```python
from build123d import *

# Parameters (mm, degrees)
CUT_EXTRUDE1_DEPTH       = 31.174758882
BOSS_EXTRUDE1_START      = 13.11
BOSS_EXTRUDE1_OUTLINE_R  = 7.478502705
BOSS_EXTRUDE1_DEPTH      = 10.08
CIRPATTERN1_COUNT        = 3
BOSS_EXTRUDE2_DEPTH      = 10.08
BOSS_EXTRUDE2_DEPTH_BACK = 495
SKETCH6_R                = 12.5


# Read off the part's stored shape, not the designer's step: Boss-Extrude1, Revolve3
with BuildPart() as part:
    # Sketch1 → Revolve1 (revolve)
    with BuildSketch(Plane.XY):
        with BuildLine():
            Line((-9.722222222, 14.550889837), (-9.722222222, 12.5))
            Line((-9.722222222, 12.5), (7.540919832, 12.5))
            Line((7.540919832, 12.5), (7.540919832, 15.791913376))
            ThreePointArc((7.540919832, 15.791913376), (-1.254812689, 17.454954744), (-9.722222222, 14.550889837))
        make_face()
    revolve(axis=Axis((-47.061566383, 0, 0), (1, 0, 0)))

    # Sketch2 → Cut-Extrude1 (cut, symmetric)
    with BuildSketch(Plane(origin=(7.540919832, 0, 0), x_dir=(0, 0, -1), z_dir=(1, 0, 0))):
        Polygon((-17.183661108, 13.11), (20.1337897, 13.11), (18.772985043, 23.764289573), (-17.183661108, 23.764289573), align=None)
    cut_extrude1 = extrude(amount=CUT_EXTRUDE1_DEPTH, both=True, mode=Mode.SUBTRACT)

    # Boss-Extrude1 outline → Boss-Extrude1 (add)
    with BuildSketch(Plane(origin=(0, 0, 0), x_dir=(1, 0, 0), z_dir=(0, 1, 0)).offset(BOSS_EXTRUDE1_START)):
        Circle(BOSS_EXTRUDE1_OUTLINE_R)
    boss_extrude1 = extrude(amount=BOSS_EXTRUDE1_DEPTH)

    # Sketch4 → Revolve2 (revolve)
    with BuildSketch(Plane(origin=(0, 0, 0), x_dir=(0, 0, -1), z_dir=(1, 0, 0)), mode=Mode.PRIVATE) as revolve2_sk:
        with BuildLine():
            Line((7.478502705, 25.422863672), (7.478502705, 23.19))
            Line((7.478502705, 23.19), (0, 23.19))
            Line((0, 23.19), (0, 26.5))
            ThreePointArc((0, 26.5), (3.777837522, 26.229333649), (7.478502705, 25.422863672))
        make_face()
    revolve2 = revolve(revolve2_sk.sketch.rotate(Axis((0, 0, 0), (0, 1, 0)), 180), axis=Axis((0, 0, 0), (0, 1, 0)))

    # Revolve3 outline → Revolve3 (revolve)
    with BuildSketch(Plane.XY):
        with BuildLine():
            Line((7.478502705, 23.190000012), (7.478502705, 13.109999988))
            Line((7.478502705, 13.109999988), (12.254015665, 13.109999994))
            ThreePointArc((12.254015665, 13.109999994), (13.25, 18.15), (12.254015665, 23.190000006))
            Line((12.254015665, 23.190000006), (7.478502705, 23.190000012))
        make_face()
    revolve3 = revolve(axis=Axis((0, 0, 0), (0, 1, 0)))

    # CirPattern1: Cut-Extrude1, Boss-Extrude1, Revolve2, Revolve3 ×3 about axis
    cirpattern1_axis = Axis((0, 0, 0), (1, 0, 0))
    add([cut_extrude1.rotate(cirpattern1_axis, i * 360 / CIRPATTERN1_COUNT) for i in range(1, CIRPATTERN1_COUNT)], mode=Mode.SUBTRACT)
    add([boss_extrude1.rotate(cirpattern1_axis, i * 360 / CIRPATTERN1_COUNT) for i in range(1, CIRPATTERN1_COUNT)])
    add([revolve2.rotate(cirpattern1_axis, i * 360 / CIRPATTERN1_COUNT) for i in range(1, CIRPATTERN1_COUNT)])
    add([revolve3.rotate(cirpattern1_axis, i * 360 / CIRPATTERN1_COUNT) for i in range(1, CIRPATTERN1_COUNT)])

    # Sketch6 → Boss-Extrude2 (add, two sides: drawn at the far end of the back side and taken through both)
    with BuildSketch(Plane.ZY.offset(9.722222222).offset(-BOSS_EXTRUDE2_DEPTH_BACK)):
        Circle(SKETCH6_R)
    extrude(amount=BOSS_EXTRUDE2_DEPTH + BOSS_EXTRUDE2_DEPTH_BACK)


solid = part.part
```
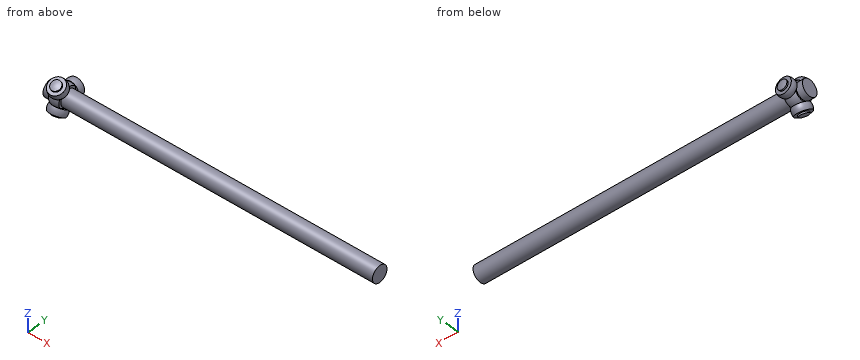
For this review, take the finished solid that the model builds, in its own axes (mm). Coordinates: 2 decimals unless noted, no trailing zeros. Loops run counter-clockwise (first coordinate to the right, second up) from the corner with the lowest first, then second, coordinate; pieces in that order, holes last.
1. Add section A-A, the plane z = 0. Give the boundary of the cut face in (x, y).
2. Add section C-C, the plane x = 108. Give the boundary of the cut face in (y, z), then the cut area to 3 significant figures.
3. Insertion check: P1, Ø1.5, axis at x = 154.5, z = 1, coming from the +Y side; P2, Ø5, axis at x = 230.5, z = -10, coming from the -Y side; P3, Ø8, axis at y = 19.5, z = 13, coming from the -X side. Each pin has a flat end and moves straight along its axis. Give the tip position at first contact, or say it passes through.
4. For line 1 (X direction, y = -12, z = -11.5); line 2 (Z direction, x = 236.5, y = -2); line 3 (X direction, y = 12, z = -4), list the stretches that pass through material, from the lowest coordinate up.
Result:
1. outline: (-19.8, -12.5) - (-9.72, -12.5) - (-9.72, -14.55) arc R17.5 ccw to (7.54, -15.79) - (7.54, -12.5) - (485.28, -12.5) - (485.28, 12.5) - (7.54, 12.5) - (7.54, 13.11) - (12.25, 13.11) arc R13.25 ccw to (12.25, 23.19) - (7.48, 23.19) - (7.48, 25.42) arc R26.5 ccw to (-7.48, 25.42) - (-7.48, 23.19) - (-12.25, 23.19) arc R13.25 ccw to (-12.25, 13.11) - (-9.72, 13.11) - (-9.72, 12.5) - (-19.8, 12.5) - close
2. outline: circle Ø25 at (0, 0)
2. area: 491 mm2
3. P1: stops at y = 12.5
3. P2: stops at y = -10
3. P3: stops at x = -9.66
4. line 1: x = -12.22 to 12.22
4. line 2: z = -12.34 to 12.34
4. line 3: x = -9.72 to 7.54
